Read the model definition and answer for the solid it produces. Units are mm, in the model's axes. A direction names the side the tool comes from. Coordinates: 2 decimals unless noted, no trailing zeros. Order: outer loops, then holes, each group sorted by start corner. A loop starts at its lowest first (then second) coordinate and runs counter-clockwise, first axis right, second up. Notation, with made-up numbers: M 34,80 L 87,80 A27 cw 87,117 Z; hole C 0,-8.75 d10. An arc over 180 degrees is marked long. Put each result on its own line as item: value.
from build123d import *

# Parameters (mm, degrees)
F1_DEPTH = 1100


# Not quite as in the source:
# - a feature names something its author has since deleted; it is built from what else it names


with BuildPart() as f1:
    # F0 (on Front) → F1 (new body)
    with BuildSketch(Plane.XZ):
        Polygon((-15.4624978453, 35.3617481887), (-30.4624978453, 35.3617481887), (-30.4624978453, 33.3617481887), (-13.4624978453, 33.3617481887), (-13.4624978453, 53.3617481887), (7.5375021547, 53.3617481887), (7.5375021547, -444.6382518113), (9.5375021547, -444.6382518113), (9.5375021547, 55.3617481887), (-15.4624978453, 55.3617481887), align=None)
    extrude(amount=F1_DEPTH)


solid = f1.part
Q1. Find section B-B on z = -132.5. Write down the section's boundary in (x, y), plus the area to 3 significant figures.
Answers below:
outline: M 7.54,-1100 L 9.54,-1100 L 9.54,0 L 7.54,0 Z
area: 2,200 mm^2
Q2. Find section A-A on y = -938. Write down the section's boundary in (x, z), plus the area to 3 significant figures.
Answers below:
outline: M -30.46,33.36 L -13.46,33.36 L -13.46,53.36 L 7.54,53.36 L 7.54,-444.64 L 9.54,-444.64 L 9.54,55.36 L -15.46,55.36 L -15.46,35.36 L -30.46,35.36 Z
area: 1,120 mm^2
Q3. Consider line 1 along X through (y, z) = (-492, -141); line 2 along Z through (x, y) = (1.5, -795.5); line 3 along Z through (x, y) = (-16, -658). Determine where each line is inside the solid, lowest interval first.
Answers below:
line 1: x = 7.54 to 9.54
line 2: z = 53.36 to 55.36
line 3: z = 33.36 to 35.36
Q4. For a pull along X with two mould halves and no side action, classify faces 1 (the face through (-3, -542, 55.362)), 2 (the face through (-15.462, -542, 46)), 3 (the face through (-3, -542, 53.362)), 4 (the face through (9.538, -542, -198)) as +X half, -X half, draft (parallel to the pull), parting line (faces both ways), or undercut.
Answers below:
face 1: draft
face 2: -X half
face 3: undercut
face 4: +X half
Q5. Given pin 1 (6.5 mm diameter, centred on x = -7, y = -715.5, fed in from -Z); pin 2 (6 mm diameter, centred on y = -394.5, z = 47.5, fed in from -X); pin 3 (4.5 mm diameter, centred on x = -19.5, y = -700, fed in from +Z), each flat-ended and moving along its own axis, determine where each tip first touches the part or whether it passes through.
Answers below:
pin 1: stops at z = 53.36
pin 2: stops at x = -15.46
pin 3: stops at z = 35.36
Q6. A tool of negligible diameter and unlimited length cuts with its end or side. For faces 5 (the face through (9, -1100, -175)), 6 (the face through (-13.462, -542, 43)), from which of +Z, -Z, +X, -X, +Y, -Y can it reach the whole face along a straight path? Write none if from no direction.
Answers below:
face 5: +Z, -Z, +X, -X, -Y
face 6: -Z, +Y, -Y
